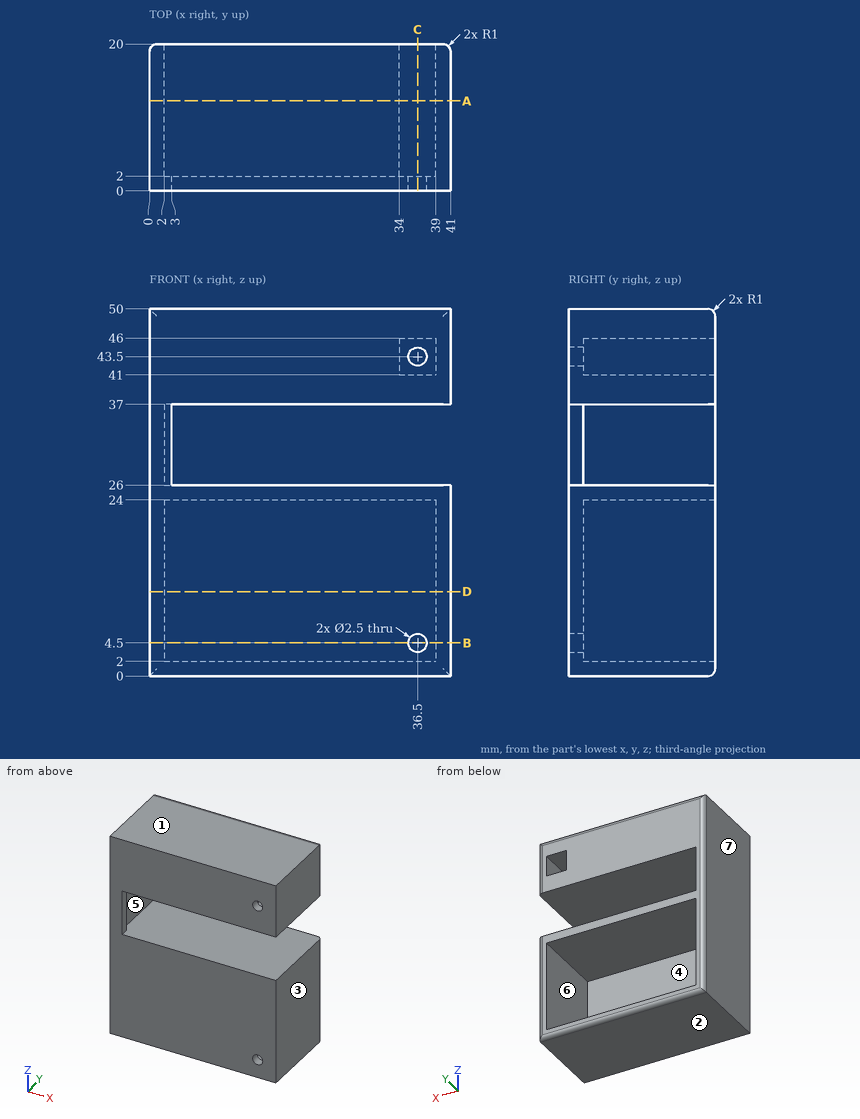
Can you work these out from the drawing? Everything is in mm from the part's minimum corner. A direction names the side the tool comes from. Give positions to 0.01 mm unless a question says otherwise; leave off trailing zeros. Loops run counter-clockwise (first coordinate to the right, second up) from the corner with the lowest first, then second, coordinate; pieces in that order, holes last. Notation, with made-up numbers: (50.25, -19) -> (95.25, -19) arc R22 cw to (95.25, 10) -> close; hole circle Ø8 at (3, -7.75). An arc over 180 degrees is marked (long way). Return JSON: item names as keys, results as strings.
Item 1: Which directions (+Z, -Z, +X, -X, +Y, -Y) give clear straight access to the entire face, cutting with the end or side of a thin tool? Please do the marked faces 5, 6 and 7.
Geometry results:
{"face 5": "+X, +Y", "face 6": "+Y", "face 7": "+Z, -Z, -X, +Y, -Y"}
Item 2: I'm going to push flat-ended pins straight in: pin 1 (2 mm diameter, centred on y = 3.5, z = 34.5, fed in from +X); pin 2 (3 mm diameter, centred on x = 31, z = 8.5, fed in from +Y); pin 3 (1 mm diameter, centred on y = 1.5, z = 29.5, fed in from +X). Where does each tip first touch, or does it pass through?
Geometry results:
{"pin 1": "stops at x = 2", "pin 2": "stops at y = 2", "pin 3": "stops at x = 3"}
Item 3: If we section it at A-A on y = 12.25: List the corners of the cut face in (x, z) for me, plus the area to 3 significant figures.
Geometry results:
{"outline": "(0, 0) -> (41, 0) -> (41, 26) -> (2, 26) -> (2, 37) -> (41, 37) -> (41, 50) -> (0, 50) -> close; hole (2, 2) -> (39, 2) -> (39, 24) -> (2, 24) -> close; hole (34, 41) -> (39, 41) -> (39, 46) -> (34, 46) -> close", "area": "782 mm²"}
Item 4: If we section it at B-B on z = 4.5: List the corners of the cut face in (x, y) for me, plus the area to 3 significant figures.
Geometry results:
{"outline": "(0, 0) -> (35.25, 0) -> (35.25, 2) -> (2, 2) -> (2, 20) -> (1, 20) arc R1 ccw to (0, 19) -> close; (37.75, 0) -> (41, 0) -> (41, 19) arc R1 ccw to (40, 20) -> (39, 20) -> (39, 2) -> (37.75, 2) -> close", "area": "149 mm²"}
Item 5: If we section it at C-C on x = 36.5: List the corners of the cut face in (y, z) for me.
Geometry results:
{"outline": "(0, 0) -> (19, 0) arc R1 ccw to (20, 1) -> (20, 2) -> (2, 2) -> (2, 3.25) -> (0, 3.25) -> close; (0, 5.75) -> (2, 5.75) -> (2, 24) -> (20, 24) -> (20, 26) -> (0, 26) -> close; (0, 37) -> (20, 37) -> (20, 41) -> (2, 41) -> (2, 42.25) -> (0, 42.25) -> close; (0, 44.75) -> (2, 44.75) -> (2, 46) -> (20, 46) -> (20, 49) arc R1 ccw to (19, 50) -> (0, 50) -> close"}
Item 6: I need wall thicknesses on L1, parallel to Z at x = 38.5, y = 18; L2, parallel to Z at x = 16.5, y = 18; L3, parallel to X at y = 4.5, z = 9. Which ranges of each line are inside material? Lowest first, please. Write a range as from..to.
Geometry results:
{"L1": "z = 0..2, 24..26, 37..41, 46..50", "L2": "z = 0..2, 24..26, 37..50", "L3": "x = 0..2, 39..41"}
Item 7: If we section it at D-D on z = 11.5: List the corners of the cut face in (x, y) for me, plus the area to 3 significant figures.
Geometry results:
{"outline": "(0, 0) -> (41, 0) -> (41, 19) arc R1 ccw to (40, 20) -> (39, 20) -> (39, 2) -> (2, 2) -> (2, 20) -> (1, 20) arc R1 ccw to (0, 19) -> close", "area": "154 mm²"}
Item 8: We'd pull the mould along Z, two halves only. Please class the marked faces 1, 2, 3 and 4: +Z half, -Z half, draft (parallel to the pull), parting line (faces both ways), or undercut.
Geometry results:
{"face 1": "+Z half", "face 2": "-Z half", "face 3": "draft", "face 4": "undercut"}
